Check sheet for the modelled part. Datum: model origin and axes. Units: mm. Face numbers are marked on the shaded views. A direction names the side the tool comes from. Coordinates: 2 decimals unless noted, no trailing zeros. Write each loop counter-clockwise with the first axis right and the second up, starting at its lowest first coordinate (ties: lowest second). Pieces come first, ordered by that corner, then holes. Notation, with made-up numbers: (65, 20.5) - (97, 20.5) arc R17 ccw to (97, 43.5) - close; hole circle Ø8 at (-16, -8). An arc over 180 degrees is marked (long way). Answer as CSV lines item,"result". Start each with the question number.
from build123d import *

# Parameters (mm, degrees)
SKETCH1_R                                           = 12
BOSS_EXTRUDE1_DEPTH                                 = 30
CSK_FOR_M5_COUNTERSUNK_FLAT_HEAD_SCREW1_D           = 5.5
CSK_FOR_M5_COUNTERSUNK_FLAT_HEAD_SCREW1_DEPTH       = 12
CSK_FOR_M5_COUNTERSUNK_FLAT_HEAD_SCREW1_CSINK_D     = 10.4
CSK_FOR_M5_COUNTERSUNK_FLAT_HEAD_SCREW1_CSINK_ANGLE = 90
CSK_FOR_M5_COUNTERSUNK_FLAT_HEAD_SCREW1_TIP         = 1.652366702
F_8_0MM_DOWEL_HOLE1_D                               = 8
F_8_0MM_DOWEL_HOLE1_DEPTH                           = 12
F_8_0MM_DOWEL_HOLE1_TIP                             = 2.403442476


with BuildPart() as part:
    # Sketch1 → Boss-Extrude1 (new body)
    with BuildSketch(Plane(origin=(0, 0, 0), x_dir=(1, 0, 0), z_dir=(0, 1, 0))):
        with Locations(Location((0, 0, 0), (0, 0, 270))):
            Circle(SKETCH1_R)
    extrude(amount=BOSS_EXTRUDE1_DEPTH)

    # CSK for M5 Countersunk Flat Head Screw1
    with Locations(Plane(origin=(0, 30, 0), x_dir=(1, 0, 0), z_dir=(0, 1, 0))):
        with Locations((0, 0)):
            CounterSinkHole(CSK_FOR_M5_COUNTERSUNK_FLAT_HEAD_SCREW1_D / 2, CSK_FOR_M5_COUNTERSUNK_FLAT_HEAD_SCREW1_CSINK_D / 2, depth=CSK_FOR_M5_COUNTERSUNK_FLAT_HEAD_SCREW1_DEPTH, counter_sink_angle=CSK_FOR_M5_COUNTERSUNK_FLAT_HEAD_SCREW1_CSINK_ANGLE)
            with Locations((0, 0, -(CSK_FOR_M5_COUNTERSUNK_FLAT_HEAD_SCREW1_DEPTH + CSK_FOR_M5_COUNTERSUNK_FLAT_HEAD_SCREW1_TIP / 2))):  # 118° drill point
                Cone(0, CSK_FOR_M5_COUNTERSUNK_FLAT_HEAD_SCREW1_D / 2, CSK_FOR_M5_COUNTERSUNK_FLAT_HEAD_SCREW1_TIP, mode=Mode.SUBTRACT)

    # Ø8.0mm Dowel Hole1
    with Locations(Plane(origin=(0, 0, 0), x_dir=(-1, 0, 0), z_dir=(0, -1, 0))):
        with Locations((0, 0)):
            Hole(F_8_0MM_DOWEL_HOLE1_D / 2, depth=F_8_0MM_DOWEL_HOLE1_DEPTH)
            with Locations((0, 0, -(F_8_0MM_DOWEL_HOLE1_DEPTH + F_8_0MM_DOWEL_HOLE1_TIP / 2))):  # 118° drill point
                Cone(0, F_8_0MM_DOWEL_HOLE1_D / 2, F_8_0MM_DOWEL_HOLE1_TIP, mode=Mode.SUBTRACT)


solid = part.part
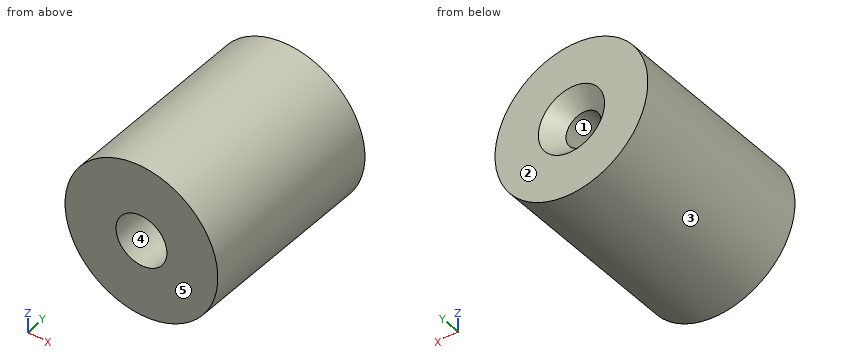
(1) Cross-section at B-B on x = -8.25. Record the boundary of the cut face in (y, z), plus the area to 3 significant figures.
(2) Go/stop test with flat-tipped pins: P1, Ø6, axis at x = -5, y = 10.5, coming from the -Z side; P2, Ø4, axis at y = 15, z = -4, coming from the +X side; P3, Ø3, axis at y = 20.5, z = -3, coming from the +X side. Record where each tip stops, or that it passes through.
(3) Cross-section at D-D on y = 2. Record the boundary of the cut face in (x, z).
(4) Cross-section at A-A on y = 20.75. Record the boundary of the cut face in (x, z), plus the area to 3 significant figures.
(5) Material ranges on probe 1 along Z at (x, y) = (1.5, 10.25); probe 2 along X at (y, z) = (13, 1.5); probe 3 along Z at (x, y) = (-9, 12.25), recorded low to high. Write a range as from..to.
(6) Release check for a two-part mould opening along X. For the marked faces 1, 2 and 3 record: pulls with the +X half, pulls with the -X half, needs draft (parallel to the pull), parting line crosses it, or undercut.
(7) Tool access check on the marked faces 4 and 5. Record the directions out of +Z, -Z, +X, -X, +Y, -Y that give a thin tool (end or side, any length) a straight path to the whole face; none if there is none.
(8) Cross-section at C-C on z = 9.25. Record the boundary of the cut face in (x, y).
Checked values:
1,outline,"(0, -8.71) - (30, -8.71) - (30, 8.71) - (0, 8.71) - close"
1,area,"523 mm^2"
2,P1,"z = -11.83"
2,P2,"x = 11.83"
2,P3,"x = 11.91"
3,outline,"circle Ø24 at (0, 0); hole circle Ø8 at (0, 0)"
4,outline,"circle Ø24 at (0, 0); hole circle Ø5.5 at (0, 0)"
4,area,"429 mm^2"
5,probe 1,"-11.91..-3.71, 3.71..11.91"
5,probe 2,"-11.91..-1.79, 1.79..11.91"
5,probe 3,"-7.94..7.94"
6,face 1,"undercut"
6,face 2,"needs draft"
6,face 3,"parting line crosses it"
7,face 4,"-Y"
7,face 5,"+Z, -Z, +X, -X, -Y"
8,outline,"(-7.64, 0) - (7.64, 0) - (7.64, 30) - (-7.64, 30) - close"
